Source: CAD feature listing. Evaluate the final solid. Frame: model axes, mm. A direction names the side the tool comes from. Round coordinates to 2 decimals unless told otherwise and drop trailing zeros. Write each loop counter-clockwise with the first axis right and the second up, starting at its lowest first coordinate (ties: lowest second). Pieces come first, ordered by that corner, then holes. Notation, with made-up numbers: (32, -21) -> (37, -21) arc R23 cw to (37, -7) -> close; hole circle Ø2 at (-26.5, 53.25). An arc over 180 degrees is marked (long way). Put each result on its own line as item: value.
```python
from build123d import *

# Parameters (mm, degrees)
F0_R     = 1
F1_DEPTH = 1.2


with BuildPart() as f1:
    # F0 (on Front) → F1 (new body)
    with BuildSketch(Plane.XZ):
        with BuildLine():
            ThreePointArc((1.5, 9.1275681318), (7.0511523881, 5.9869650074), (9.25, 0))
            ThreePointArc((9.25, 0), (-5.9869650074, -7.0511523881), (-1.5, 9.1275681318))
            Line((-1.5, 9.1275681318), (-4.4093787034, 9.1275681318))
            ThreePointArc((-4.4093787034, 9.1275681318), (-6.0206658379, -10.156062289), (11, -0.95))
            ThreePointArc((11, -0.95), (9.206062289, 5.0706658379), (4.4093787034, 9.1275681318))
            Line((4.4093787034, 9.1275681318), (1.5, 9.1275681318))
        make_face()
        with BuildLine():
            Line((-4.5, 9.1275681318), (-4.4093787034, 9.1275681318))
            ThreePointArc((-4.4093787034, 9.1275681318), (-2.9829779875, 9.6378157486), (-1.5, 9.9472473589))
            Line((-1.5, 9.9472473589), (-1.5, 13.0275681318))
            Line((-1.5, 13.0275681318), (-4.5, 13.0275681318))
            Line((-4.5, 13.0275681318), (-4.5, 9.1275681318))
        make_face()
        with Locations((-3, 11.1275681318)):
            Circle(F0_R, mode=Mode.SUBTRACT)
        with BuildLine():
            Line((-4.4093787034, 9.1275681318), (-1.5, 9.1275681318))
            Line((-1.5, 9.1275681318), (-1.5, 9.9472473589))
            ThreePointArc((-1.5, 9.9472473589), (-2.9829779875, 9.6378157486), (-4.4093787034, 9.1275681318))
        make_face()
        with BuildLine():
            ThreePointArc((1.5, 9.9472473589), (2.9829779875, 9.6378157486), (4.4093787034, 9.1275681318))
            Line((4.4093787034, 9.1275681318), (4.5, 9.1275681318))
            Line((4.5, 9.1275681318), (4.5, 13.0275681318))
            Line((4.5, 13.0275681318), (1.5, 13.0275681318))
            Line((1.5, 13.0275681318), (1.5, 9.9472473589))
        make_face()
        with Locations((3, 11.1275681318)):
            Circle(F0_R, mode=Mode.SUBTRACT)
        with BuildLine():
            Line((1.5, 9.9472473589), (1.5, 9.1275681318))
            Line((1.5, 9.1275681318), (4.4093787034, 9.1275681318))
            ThreePointArc((4.4093787034, 9.1275681318), (2.9829779875, 9.6378157486), (1.5, 9.9472473589))
        make_face()
    extrude(amount=F1_DEPTH)


solid = f1.part
```
Q1. Draft query along Z for faces 4 (the flat face through (-3, -1, 13.028)), 5 (the cylindrical face through (2.783, -0.592, 10.151)), 6 (the cylindrical face through (-3.217, -0.592, 10.151)), 7 (the flat face through (1.5, -1, 11)). Return one class per face: +Z half, -Z half, draft (parallel to the pull), parting line (faces both ways), or undercut.
Ans:
face 4: +Z half
face 5: undercut
face 6: undercut
face 7: draft
Q2. Cut plane A-A on z = -7.5. Output: boundary loops of the cut face in (x, y).
Ans:
outline: (-8.84, -1.2) -> (-5.41, -1.2) -> (-5.41, 0) -> (-8.84, 0) -> close; (5.41, -1.2) -> (8.84, -1.2) -> (8.84, 0) -> (5.41, 0) -> close
Q3. Cut plane B-B on x = -5.5. Output: boundary loops of the cut face in (y, z), and give its area (3 significant figures).
Ans:
outline: (-1.2, -10.48) -> (0, -10.48) -> (0, -7.44) -> (-1.2, -7.44) -> close; (-1.2, 7.44) -> (0, 7.44) -> (0, 8.58) -> (-1.2, 8.58) -> close
area: 5.01 mm^2
Q4. Reachability of faces 1 (the flat face through (4.5, -1, 11)), 2 (the flat face through (-1.5, -1, 11)), 3 (the flat face through (-4.5, -1, 11)) from +Z, -Z, +X, -X, +Y, -Y: full face, straight path, thin tool, end or side. Return the list, or none.
Ans:
face 1: +Z, +X, +Y, -Y
face 2: +Z, +Y, -Y
face 3: +Z, -X, +Y, -Y
Q5. Cut plane C-C on y = -0.55. Output: boundary loops of the cut face in (x, z).
Ans:
outline: (-4.5, 9.13) -> (-4.41, 9.13) arc R11 ccw (long way) to (4.41, 9.13) -> (4.5, 9.13) -> (4.5, 13.03) -> (1.5, 13.03) -> (1.5, 9.13) arc R9.25 cw (long way) to (-1.5, 9.13) -> (-1.5, 13.03) -> (-4.5, 13.03) -> close; hole circle Ø2 at (-3, 11.13); hole circle Ø2 at (3, 11.13)
Q6. Material intervals for line 1 (Z direction, x = 3, y = -0.3); line 2 (Z direction, x = 0, y = -0.3); line 3 (X direction, y = -0.95, z = 11.75), sorted ascending. Write a range as [from, to].
Ans:
line 1: z = [-11.53, -8.75], [8.75, 10.13], [12.13, 13.03]
line 2: z = [-11.95, -9.25]
line 3: x = [-4.5, -3.78], [-2.22, -1.5], [1.5, 2.22], [3.78, 4.5]
Q7. Cut plane D-D on x = -3. Output: boundary loops of the cut face in (y, z).
Ans:
outline: (-1.2, -11.53) -> (0, -11.53) -> (0, -8.75) -> (-1.2, -8.75) -> close; (-1.2, 8.75) -> (0, 8.75) -> (0, 10.13) -> (-1.2, 10.13) -> close; (-1.2, 12.13) -> (0, 12.13) -> (0, 13.03) -> (-1.2, 13.03) -> close
